from build123d import *

# Parameters (mm, degrees)
SKETCH1_R           = 12.6746
SKETCH1_R_2         = 4.0005
SKETCH1_R_3         = 1.1938
BOSS_EXTRUDE1_DEPTH = 6.35
CHAMFER1_SIZE       = 0.254


with BuildPart() as part:
    # Sketch1 → Boss-Extrude1 (new body)
    with BuildSketch(Plane(origin=(0, 0, 0), x_dir=(1, 0, 0), z_dir=(0, 1, 0))):
        with Locations(Location((0, 0, 0), (0, 0, 270))):
            Circle(SKETCH1_R)
        with Locations(Location((0, 0, 0), (0, 0, 270))):
            Circle(SKETCH1_R_2, mode=Mode.SUBTRACT)
        with Locations(Location((0, 8.3312, 0), (0, 0, 270))):
            Circle(SKETCH1_R_3, mode=Mode.SUBTRACT)
        with Locations(Location((8.3312, 0, 0), (0, 0, 270))):
            Circle(SKETCH1_R_3, mode=Mode.SUBTRACT)
        with Locations(Location((0, -8.3312, 0), (0, 0, 270))):
            Circle(SKETCH1_R_3, mode=Mode.SUBTRACT)
        with Locations(Location((-8.3312, 0, 0), (0, 0, 270))):
            Circle(SKETCH1_R_3, mode=Mode.SUBTRACT)
        with Locations(Location((-5.756293352, 6.022788415, 0), (0, 0, 270))):
            Circle(SKETCH1_R_3, mode=Mode.SUBTRACT)
        with Locations(Location((6.022788415, 5.756293352, 0), (0, 0, 270))):
            Circle(SKETCH1_R_3, mode=Mode.SUBTRACT)
        with Locations(Location((6.022788415, -5.756293352, 0), (0, 0, 270))):
            Circle(SKETCH1_R_3, mode=Mode.SUBTRACT)
        with Locations(Location((-5.756293352, -6.022788415, 0), (0, 0, 270))):
            Circle(SKETCH1_R_3, mode=Mode.SUBTRACT)
    extrude(amount=BOSS_EXTRUDE1_DEPTH)

    # Chamfer1
    chamfer1_edges = [part.edges().sort_by_distance(p)[0] for p in [
        (8.3312, 0, -1.1938),
        (8.3312, 6.35, -1.1938),
        (0, 0, 7.1374),
        (0, 6.35, 7.1374),
        (0, 0, -12.6746),
        (-8.3312, 0, -1.1938),
        (-8.3312, 6.35, -1.1938),
        (-5.756293352, 0, -7.216588415),
        (-5.756293352, 6.35, -7.216588415),
        (6.022788415, 0, -6.950093352),
        (6.022788415, 6.35, -6.950093352),
        (6.022788415, 0, 4.562493352),
        (6.022788415, 6.35, 4.562493352),
        (-5.756293352, 0, 4.828988415),
        (-5.756293352, 6.35, 4.828988415),
        (0, 6.35, -12.6746),
        (0, 0, -4.0005),
        (0, 6.35, -4.0005),
        (0, 0, -9.525),
        (0, 6.35, -9.525),
    ]]
    chamfer(chamfer1_edges, length=CHAMFER1_SIZE)


solid = part.part
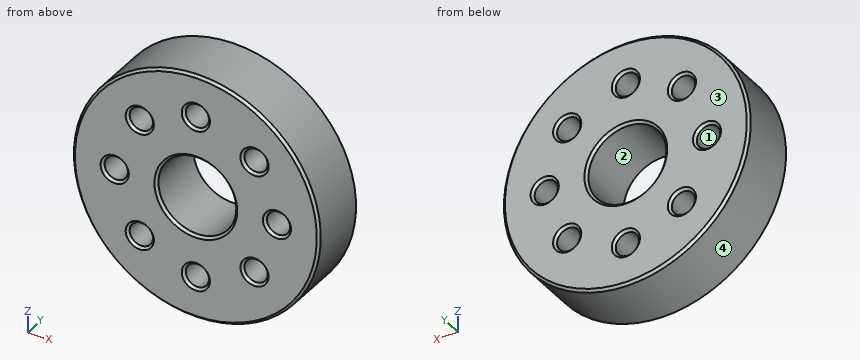
Geometry check sheet. Reference: the model listing, model coordinates, mm. Face numbers are marked on the shaded views. Round coordinates to 2 decimals unless told otherwise and drop trailing zeros. One line per item, written item: value.
1. Mould release check, pull along X, two halves, no side actions. Record for the marked faces 1, 2, 3 and 4: released by +X, released by -X, zero draft, split by the parting line, or undercut.
The answers:
face 1: undercut
face 2: undercut
face 3: zero draft
face 4: split by the parting line
2. Cross-section at A-A on z = 0. Give the number of separate pieces and of enclosed holes in the cut face, and give its area (3 significant figures).
The answers:
separate pieces: 4
enclosed holes: 0
area: 79.3 mm^2
3. Depth check by flat-ended pin: pin 1 Ø1 at (y, z) = (4.5, 4.5) entering from +X; pin 2 Ø1 at (y, z) = (4.5, -7.5) entering from +X. Enter the tip coordinate at first touch or a pass-through.
The answers:
pin 1: stops at x = 12.03
pin 2: stops at x = 10.57
4. Scan lines: L1, parallel to X at y = 3.5, z = 0 (1 decimal); L2, parallel to X at y = 1.25, z = -1; L3, parallel to Z at x = -5, y = 5.5. Record each from-to range of solid material in increasing order.
The answers:
L1: x = -12.7 to -9.5, -7.1 to -4, 4 to 7.1, 9.5 to 12.7
L2: x = -12.64 to -8.98, -7.68 to -3.87, 3.87 to 7.68, 8.98 to 12.64
L3: z = -11.65 to -6.95, -5.1 to 5.1, 6.95 to 11.65
